Input: dimensioned drawing with shaded views. Units: mm. Origin: part minimum x, y, z. A direction names the side the tool comes from. Give positions to 0.01 mm unless a question says otherwise; leave off trailing zeros. Order: outer loops, then holes, each group sorted by start corner. A loop starts at its lowest first (then second) coordinate and runs counter-clockwise, first axis right, second up. Notation, with made-up numbers: M -27.75,55.5 L 11.25,55.5 A8 cw 11.25,65.5 Z; hole C 27,6.25 d10. An arc over 180 degrees is marked long. Answer in a Markdown table with one row per item. Add a question column.
(1) Section query D-D, the plane z = 40. Return loops of the section in (x, y).
(2) Section query A-A, the plane z = 3. Return loops of the section in (x, y), plus the area to 3 significant figures.
(3) Section query C-C, the plane x = 23.5. Return loops of the section in (y, z).
(4) Mould query, pull axis X, two halves, no side actions, for the marked faces 1, 2 and 3. Classes: pulls with the +X half, pulls with the -X half, needs draft (parallel to the pull), parting line crosses it, or undercut.
(5) Set-up query: the marked faces 4, 5 and 6. Return all of +Z, -Z, +X, -X, +Y, -Y with unobstructed straight access to the full face (end or side cutting, diameter ignored); none if empty.
(6) Section query B-B, the plane x = 39. Return loops of the section in (y, z), plus the area to 3 significant figures.
(7) Pin query (flat end, axial travel): P1, Ø2, axis at x = 39, z = 48, coming from the +Y side; P2, Ø9, axis at x = 44, y = 4, coming from the -Z side; P3, Ø8, axis at x = 40.5, y = 4.5, coming from the +Z side; P4, Ø1, axis at x = 9, z = 25.5, coming from the +Y side. Return the tip coordinate at first contact, or that it passes through.
(8) Material intervals for line 1 along X through (y, z) = (19, 48); line 2 along X through (y, z) = (19.5, 55); line 3 along Y through (x, z) = (4, 28), sorted ascending.
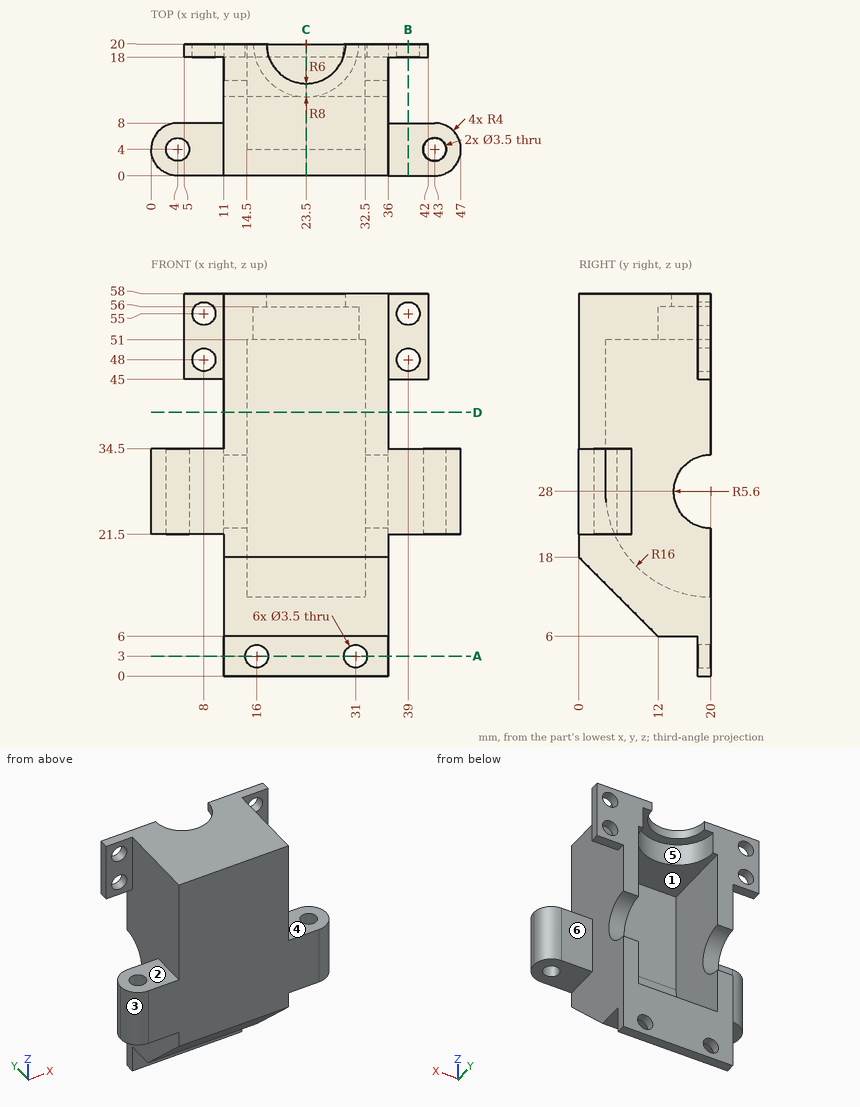
Values follow:
| question | item | result |
|---|---|---|
| 1 | outline | M 11,0 L 36,0 L 36,20 L 32.5,20 L 32.5,4 L 14.5,4 L 14.5,20 L 11,20 Z |
| 2 | outline | M 11,18 L 14.25,18 L 14.25,20 L 11,20 Z; M 17.75,18 L 29.25,18 L 29.25,20 L 17.75,20 Z; M 32.75,18 L 36,18 L 36,20 L 32.75,20 Z |
| 2 | area | 36.0 mm² |
| 3 | outline | M 0,18 L 12,6 L 18,6 L 18,0 L 20,0 L 20,12 A16 cw 4,28 L 4,51 L 12,51 L 12,56 L 14,56 L 14,58 L 0,58 Z |
| 4 | face 1 | undercut |
| 4 | face 2 | needs draft |
| 4 | face 3 | pulls with the -X half |
| 5 | face 4 | +Z, +X, +Y, -Y |
| 5 | face 5 | +Y |
| 5 | face 6 | +Z, -Z, +X, +Y |
| 6 | outline | M 0,21.5 L 8,21.5 L 8,34.5 L 0,34.5 Z; M 18,45 L 20,45 L 20,46.25 L 18,46.25 Z; M 18,49.75 L 20,49.75 L 20,53.25 L 18,53.25 Z; M 18,56.75 L 20,56.75 L 20,58 L 18,58 Z |
| 6 | area | 116 mm² |
| 7 | P1 | passes through |
| 7 | P2 | stops at z = 21.5 |
| 7 | P3 | stops at z = 34.5 |
| 7 | P4 | stops at y = 8 |
| 8 | line 1 | x = 5 to 6.25, 9.75 to 14.5, 32.5 to 37.25, 40.75 to 42 |
| 8 | line 2 | x = 5 to 6.25, 9.75 to 15.52, 31.48 to 37.25, 40.75 to 42 |
| 8 | line 3 | y = 0 to 2.25, 5.75 to 8 |
